```python
from build123d import *

# Parameters (mm, degrees)
SKETCH1_R           = 5
BOSS_EXTRUDE1_DEPTH = 22.5
SKETCH3_W           = 10
SKETCH3_H           = 30
CUT_EXTRUDE1_DEPTH  = 45
SKETCH4_R           = 1.5
CUT_EXTRUDE2_DEPTH  = 45
SKETCH4_3_R         = 1.5
CUT_EXTRUDE3_DEPTH  = 45
SKETCH6_W           = 10
SKETCH6_H           = 30
CUT_EXTRUDE4_DEPTH  = 45
SKETCH7_W           = 12.5
SKETCH7_H           = 30
CUT_EXTRUDE5_DEPTH  = 45
SKETCH8_W           = 5
SKETCH8_H           = 10.669872981
CUT_EXTRUDE6_DEPTH  = 45
SKETCH9_R           = 1.25
CUT_EXTRUDE7_DEPTH  = 150


with BuildPart() as part:
    # Sketch1 → Boss-Extrude1 (new, symmetric)
    with BuildSketch(Plane(origin=(0, 0, 0), x_dir=(0, 0, -1), z_dir=(1, 0, 0))):
        with BuildLine():
            Line((-24, 50), (-24, 40))
            Line((-24, 40), (-30, 40))
            Line((-30, 40), (-30, 0))
            Line((-30, 0), (-30, -12))
            Line((-30, -12), (0, -12))
            Line((0, -12), (0, 0))
            Line((0, 0), (0, 40))
            Line((0, 40), (-6, 40))
            Line((-6, 40), (-6, 50))
            Line((-6, 50), (-12, 50))
            Line((-12, 50), (-12, 38.485281374))
            ThreePointArc((-12, 38.485281374), (-15, 21), (-18, 38.485281374))
            Line((-18, 38.485281374), (-18, 50))
            Line((-18, 50), (-24, 50))
        make_face()
        with Locations(Location((-15, 3, 0), (0, 0, 180))):
            Circle(SKETCH1_R, mode=Mode.SUBTRACT)
    extrude(amount=BOSS_EXTRUDE1_DEPTH, both=True)

    # Sketch3 → Cut-Extrude1 (cut)
    with BuildSketch(Plane(origin=(0, 0, 0), x_dir=(-1, 0, 0), z_dir=(0, 0, -1))):
        with Locations((17.5, 3)):
            Rectangle(SKETCH3_W, SKETCH3_H)
    extrude(amount=-CUT_EXTRUDE1_DEPTH, mode=Mode.SUBTRACT)

    # Sketch4 → Cut-Extrude2 (cut)
    with BuildSketch(Plane.ZY.offset(12.5)):
        with Locations(Location((22.5, 3, 0), (0, 0, 270))):
            Circle(SKETCH4_R)
    extrude(amount=-CUT_EXTRUDE2_DEPTH, mode=Mode.SUBTRACT)

    # Sketch4_3 → Cut-Extrude3 (cut)
    with BuildSketch(Plane.ZY.offset(12.5)):
        with Locations(Location((7.5, 3, 0), (0, 0, 270))):
            Circle(SKETCH4_3_R)
    extrude(amount=-CUT_EXTRUDE3_DEPTH, mode=Mode.SUBTRACT)

    # Sketch6 → Cut-Extrude4 (cut)
    with BuildSketch(Plane(origin=(0, 0, 0), x_dir=(-1, 0, 0), z_dir=(0, 0, -1))):
        with Locations((-5, 3)):
            Rectangle(SKETCH6_W, SKETCH6_H)
    extrude(amount=-CUT_EXTRUDE4_DEPTH, mode=Mode.SUBTRACT)

    # Sketch7 → Cut-Extrude5 (cut)
    with BuildSketch(Plane(origin=(0, 0, 0), x_dir=(-1, 0, 0), z_dir=(0, 0, -1))):
        with Locations((-16.25, 3)):
            Rectangle(SKETCH7_W, SKETCH7_H)
    extrude(amount=-CUT_EXTRUDE5_DEPTH, mode=Mode.SUBTRACT)

    # Sketch8 → Cut-Extrude6 (cut)
    with BuildSketch(Plane(origin=(0, 0, 0), x_dir=(0, 0, -1), z_dir=(1, 0, 0))):
        with Locations((-15, -6.66506351)):
            Rectangle(SKETCH8_W, SKETCH8_H)
    extrude(amount=-CUT_EXTRUDE6_DEPTH, mode=Mode.SUBTRACT)

    # Sketch9 → Cut-Extrude7 (cut)
    with BuildSketch(Plane(origin=(0, 0, 6), x_dir=(-1, 0, 0), z_dir=(0, 0, -1))):
        with Locations(Location((12.5, 45, 0), (0, 0, 90))):
            Circle(SKETCH9_R)
        with Locations(Location((-7.5, 45, 0), (0, 0, 90))):
            Circle(SKETCH9_R)
    extrude(amount=-CUT_EXTRUDE7_DEPTH, mode=Mode.SUBTRACT)


solid = part.part
```
Input: part model. Units: mm. Frame: model coordinates. A direction names the side the tool comes from. Give positions to 0.01 mm unless a question says otherwise; leave off trailing zeros. Order: outer loops, then holes, each group sorted by start corner. A loop starts at its lowest first (then second) coordinate and runs counter-clockwise, first axis right, second up.
1. Cut plane C-C (z = 22.5). Return loops of the section in (x, y).
Computed:
outline: (-22.5, 18) - (-12.5, 18) - (-12.5, 4.5) - (0, 4.5) - (0, 18) - (22.5, 18) - (22.5, 25.03) - (-22.5, 25.03) - close; (-22.5, 34.97) - (22.5, 34.97) - (22.5, 50) - (-22.5, 50) - close; (-12.5, -12) - (0, -12) - (0, 1.5) - (-12.5, 1.5) - close; hole circle Ø2.5 at (-12.5, 45); hole circle Ø2.5 at (7.5, 45)
2. Line query: probe 1 along X at (y, z) = (45, 8.35); probe 2 along Z at (x, y) = (-6, 3); probe 3 along Z at (x, y) = (-6.5, 45). Output: solid intervals per line, ascending.
Computed:
probe 1: x = -22.5 to -13.75, -11.25 to 6.25, 8.75 to 22.5
probe 2: z = 0 to 6, 9 to 10, 20 to 21, 24 to 30
probe 3: z = 6 to 12, 18 to 24
3. Cut plane D-D (x = -10.5). Return loops of the section in (y, z), and give its area (3 significant figures).
Computed:
outline: (-12, 0) - (40, 0) - (40, 6) - (50, 6) - (50, 12) - (38.49, 12) arc R9 cw (long way) to (38.49, 18) - (50, 18) - (50, 24) - (40, 24) - (40, 30) - (-12, 30) - (-12, 17.5) - (-1.33, 17.5) arc R5 cw (long way) to (-1.33, 12.5) - (-12, 12.5) - close; hole circle Ø3 at (3, 7.5); hole circle Ø3 at (3, 22.5)
area: 1,270 mm2
4. Cut plane A-A (y = 3). Return loops of the section in (x, z), and give its area (3 significant figures).
Computed:
outline: (-12.5, 0) - (0, 0) - (0, 6) - (-12.5, 6) - close; (-12.5, 9) - (0, 9) - (0, 10) - (-12.5, 10) - close; (-12.5, 20) - (0, 20) - (0, 21) - (-12.5, 21) - close; (-12.5, 24) - (0, 24) - (0, 30) - (-12.5, 30) - close
area: 175 mm2
5. Draft query along Z for faces 4 (the face through (0, 45, 24)), 5 (the face through (-22.5, 38, 22)), 6 (the face through (0, 21, 15)). Return one class per face: released by +Z, released by -Z, zero draft, split by the parting line, or undercut.
Computed:
face 4: released by +Z
face 5: zero draft
face 6: undercut
6. Set-up query: faces 1 (the face through (-6, -7, 17.5)), 2 (the face through (0, 40, 27)), 3 (the face through (-17, 18, 15)). Return all of +Z, -Z, +X, -X, +Y, -Y with unobstructed straight access to the full face (end or side cutting, diameter ignored); none if empty.
Computed:
face 1: +X, -X, -Y
face 2: +Z, +X, -X, +Y
face 3: +Z, -Z, -X, -Y
7. Pin query (flat end, axial travel): pin 1 Ø4 at (x, y) = (7.5, 45) entering from +Z; pin 2 Ø2 at (x, y) = (-12.5, 45) entering from -Z; pin 3 Ø12 at (y, z) = (13.5, 8) entering from +X; pin 4 Ø15 at (y, z) = (3.5, 12.5) entering from +X. Return the tip coordinate at first contact, or that it passes through.
Computed:
pin 1: stops at z = 24
pin 2: passes through
pin 3: stops at x = 22.5
pin 4: stops at x = 0
8. Cut plane B-B (x = 7.5). Return loops of the section in (y, z), and give its area (3 significant figures).
Computed:
outline: (18, 0) - (40, 0) - (40, 6) - (43.75, 6) - (43.75, 12) - (38.49, 12) arc R9 cw (long way) to (38.49, 18) - (43.75, 18) - (43.75, 24) - (40, 24) - (40, 30) - (18, 30) - close; (46.25, 6) - (50, 6) - (50, 12) - (46.25, 12) - close; (46.25, 18) - (50, 18) - (50, 24) - (46.25, 24) - close
area: 489 mm2
